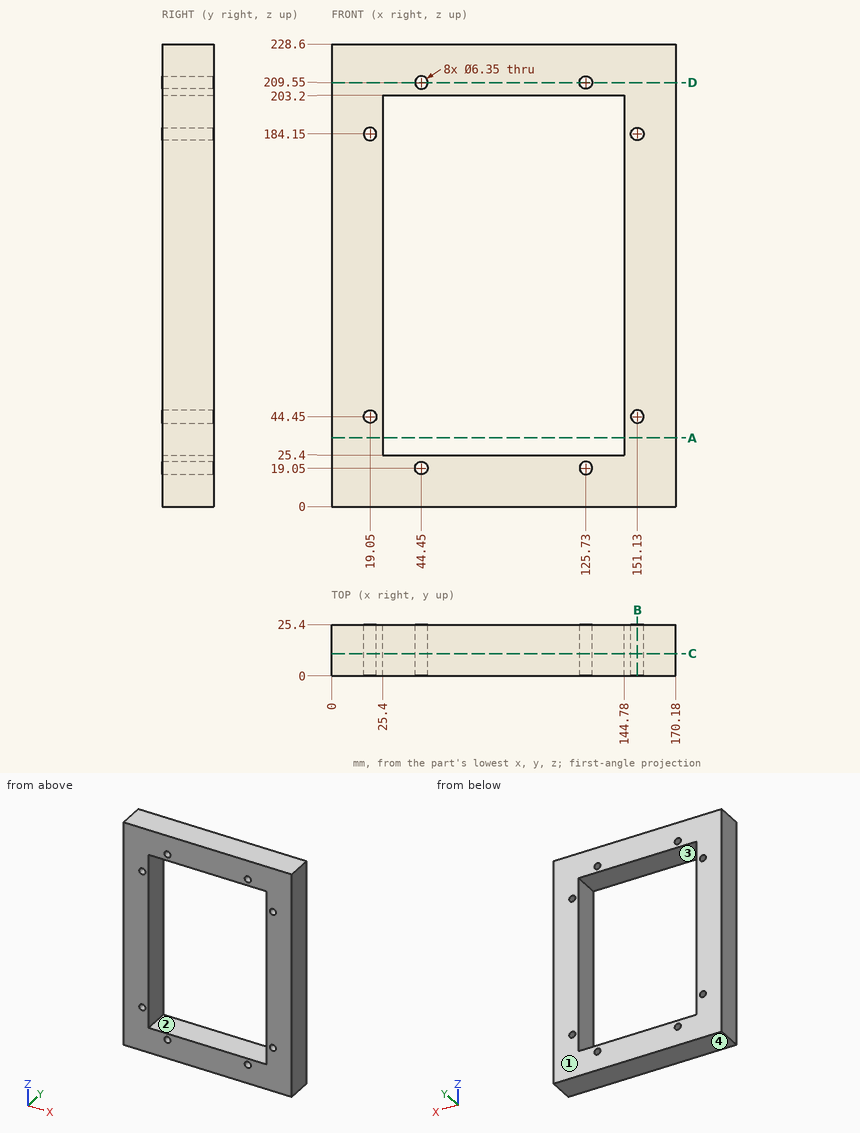
Study the drawing (mm; zero at the part's minimum x, y, z) and answer. Give positions to 0.01 mm unless a question says otherwise; leave off trailing zeros. Loops run counter-clockwise (first coordinate to the right, second up) from the corner with the lowest first, then second, coordinate; pieces in that order, holes last. Notation, with made-up numbers: M -20.75,-22.75 L 12.25,-22.75 A25 cw 12.25,0.25 Z; hole C 55,86.5 d10. An arc over 180 degrees is marked long. Answer as CSV lines item,"result".
Item 1: The part is cut by section D-D (z = 209.55). Give the vertices of the cut face in (x, y) (3 decimals), and give its area (3 significant figures).
Values follow:
outline,"M 0,0 L 41.275,0 L 41.275,25.4 L 0,25.4 Z; M 47.625,0 L 122.555,0 L 122.555,25.4 L 47.625,25.4 Z; M 128.905,0 L 170.18,0 L 170.18,25.4 L 128.905,25.4 Z"
area,"4,000 mm^2"
Item 2: Straight lines are drawn through the part: line 1 along X through (y, z) = (17.25, 19.05) (3 decimals); line 2 along Z through (x, y) = (151.13, 12.25) (3 decimals); line 3 along X through (y, z) = (20.75, 44.45) (3 decimals). For each, find the intervals that lie inside material, in ascending order. Write a range as [from, to].
Values follow:
line 1,"x = [0, 41.275], [47.625, 122.555], [128.905, 170.18]"
line 2,"z = [0, 41.275], [47.625, 180.975], [187.325, 228.6]"
line 3,"x = [0, 15.875], [22.225, 25.4], [144.78, 147.955], [154.305, 170.18]"
Item 3: The part is cut by section C-C (y = 11). Give the number of separate pieces and of enclosed holes in the cut face, and give its area (3 significant figures).
Values follow:
separate pieces,"1"
enclosed holes,"9"
area,"17,400 mm^2"
Item 4: The part is cut by section B-B (x = 151.13). Give the vertices of the cut face in (y, z) (3 decimals).
Values follow:
outline,"M 0,0 L 25.4,0 L 25.4,41.275 L 0,41.275 Z; M 0,47.625 L 25.4,47.625 L 25.4,180.975 L 0,180.975 Z; M 0,187.325 L 25.4,187.325 L 25.4,228.6 L 0,228.6 Z"
Item 5: The part is cut by section A-A (z = 34). Give the vertices of the cut face in (x, y), and give its area (3 significant figures).
Values follow:
outline,"M 0,0 L 25.4,0 L 25.4,25.4 L 0,25.4 Z; M 144.78,0 L 170.18,0 L 170.18,25.4 L 144.78,25.4 Z"
area,"1,290 mm^2"
Item 6: The mould has two halves that part along Z. Classify the marked faces 1, 2, 3 and 4: released by +Z, released by -Z, zero draft, split by the parting line, or undercut.
Values follow:
face 1,"zero draft"
face 2,"undercut"
face 3,"undercut"
face 4,"released by -Z"
Item 7: Given pin 1 Ø8.5 at (x, z) = (125.73, 209.55) entering from +Y, flat-ended and moving along its own axis, determine where the tip first touches the part or whether it passes through.
Values follow:
pin 1,"stops at y = 25.4"
